```python
from build123d import *

# Parameters (mm, degrees)
BOSS_EXTRUDE1_DEPTH = 3.175
CUT_EXTRUDE1_REACH  = 70.759
SKETCH2_R           = 1.5875
SKETCH2_R_2         = 3.302


with BuildPart() as part:
    # Sketch1 → Boss-Extrude1 (new body)
    with BuildSketch(Plane(origin=(0, 0, 0), x_dir=(1, 0, 0), z_dir=(0, 1, 0))):
        with BuildLine():
            Line((44.45, 25.4), (54.61, 25.4))
            ThreePointArc((54.61, 25.4), (56.406051224, 24.656051224), (57.15, 22.86))
            Line((57.15, 22.86), (57.15, 2.54))
            ThreePointArc((57.15, 2.54), (56.406051224, 0.743948776), (54.61, 0))
            Line((54.61, 0), (2.54, 0))
            ThreePointArc((2.54, 0), (0.743948776, 0.743948776), (0, 2.54))
            Line((0, 2.54), (0, 22.86))
            ThreePointArc((0, 22.86), (0.743948776, 24.656051224), (2.54, 25.4))
            Line((2.54, 25.4), (39.37, 25.4))
            Line((39.37, 25.4), (39.37, 36.83))
            ThreePointArc((39.37, 36.83), (39.741974388, 37.728025612), (40.64, 38.1))
            Line((40.64, 38.1), (43.18, 38.1))
            ThreePointArc((43.18, 38.1), (44.078025612, 37.728025612), (44.45, 36.83))
            Line((44.45, 36.83), (44.45, 25.4))
        make_face()
    extrude(amount=BOSS_EXTRUDE1_DEPTH)

    # Sketch2 → Cut-Extrude1 (cut, up to next)
    with BuildSketch(Plane(origin=(0, 3.175, 0), x_dir=(1, 0, 0), z_dir=(0, 1, 0)), mode=Mode.PRIVATE) as cut_extrude1_sk1:
        with Locations(Location((12.7, 12.7, 0), (0, 0, 270))):
            Circle(SKETCH2_R)
    cut_extrude1_tool1 = extrude(cut_extrude1_sk1.sketch, amount=-CUT_EXTRUDE1_REACH, mode=Mode.PRIVATE) & part.part
    # Sketch2 → Cut-Extrude1 (cut, up to next)
    with BuildSketch(Plane(origin=(0, 3.175, 0), x_dir=(1, 0, 0), z_dir=(0, 1, 0)), mode=Mode.PRIVATE) as cut_extrude1_sk2:
        with Locations(Location((26.699972, 12.7, 0), (0, 0, 270))):
            Circle(SKETCH2_R)
    cut_extrude1_tool2 = extrude(cut_extrude1_sk2.sketch, amount=-CUT_EXTRUDE1_REACH, mode=Mode.PRIVATE) & part.part
    # Sketch2 → Cut-Extrude1 (cut, up to next)
    with BuildSketch(Plane(origin=(0, 3.175, 0), x_dir=(1, 0, 0), z_dir=(0, 1, 0)), mode=Mode.PRIVATE) as cut_extrude1_sk3:
        with Locations(Location((41.91, 12.7, 0), (0, 0, 270))):
            Circle(SKETCH2_R_2)
    cut_extrude1_tool3 = extrude(cut_extrude1_sk3.sketch, amount=-CUT_EXTRUDE1_REACH, mode=Mode.PRIVATE) & part.part
    add(cut_extrude1_tool1.solids().sort_by_distance((12.7, 3.175, -12.7))[0], mode=Mode.SUBTRACT)
    add(cut_extrude1_tool2.solids().sort_by_distance((26.699972, 3.175, -12.7))[0], mode=Mode.SUBTRACT)
    add(cut_extrude1_tool3.solids().sort_by_distance((41.91, 3.175, -12.7))[0], mode=Mode.SUBTRACT)


solid = part.part
```
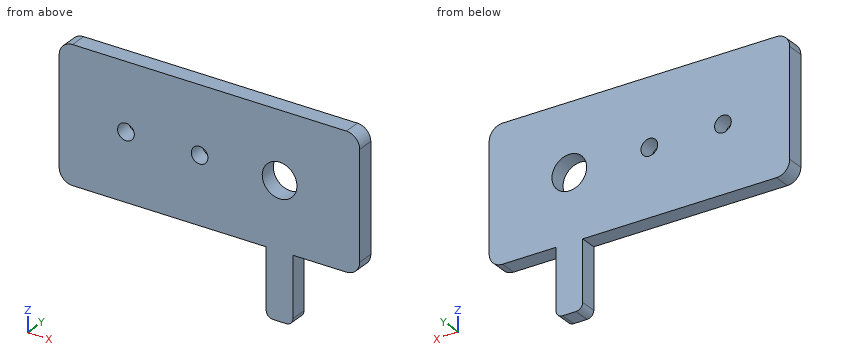
Part model, mm, in its own coordinate system. Give positions to 0.01 mm unless a question says otherwise; leave off trailing zeros. Order: outer loops, then holes, each group sorted by start corner. A loop starts at its lowest first (then second) coordinate and runs counter-clockwise, first axis right, second up. Notation, with made-up numbers: M -30.75,53.5 L 3.25,53.5 A20 ccw 3.25,73.5 Z; hole C 31.5,-29 d10. An arc over 180 degrees is marked long. Use a Markdown table: item, result. Add a question column.
(1) Drop flat-ended pins along their axis: P1, Ø2, axis at x = 37, z = -33.5, coming from the -Y side; P2, Ø1.6, axis at y = 1.5, z = -31, coming from the -X side. Give the stop position or say it passes through.
(2) Saw through at C-C, the plane x = 12.7. Give the cut face in (y, z) (1 decimal), and give its area (3 significant figures).
(3) Saw through at B-B, the plane x = 41.91. Give the cut face in (y, z) (3 decimals).
(4) Saw through at A-A, the plane z = -12.7. Give the number of separate pieces and of enclosed holes in the cut face, and give its area (3 significant figures).
(5) Probe line 1 along X through (y, z) = (1.8, -12.7); line 2 along Z through (x, y) = (28.5, 0.9); line 3 along Z through (x, y) = (39.5, 1.95). List the from-to ranges inside material, lowest first. Write a range as [from, to].
Answer key:
| question | item | result |
|---|---|---|
| 1 | P1 | through |
| 1 | P2 | x = 39.37 |
| 2 | outline | M 0,-25.4 L 3.2,-25.4 L 3.2,-14.3 L 0,-14.3 Z; M 0,-11.1 L 3.2,-11.1 L 3.2,0 L 0,0 Z |
| 2 | area | 70.6 mm^2 |
| 3 | outline | M 0,-38.1 L 3.175,-38.1 L 3.175,-16.002 L 0,-16.002 Z; M 0,-9.398 L 3.175,-9.398 L 3.175,0 L 0,0 Z |
| 4 | separate pieces | 4 |
| 4 | enclosed holes | 0 |
| 4 | area | 140 mm^2 |
| 5 | line 1 | [0, 11.11], [14.29, 25.11], [28.29, 38.61], [45.21, 57.15] |
| 5 | line 2 | [-25.4, 0] |
| 5 | line 3 | [-37.39, -14.96], [-10.44, 0] |
